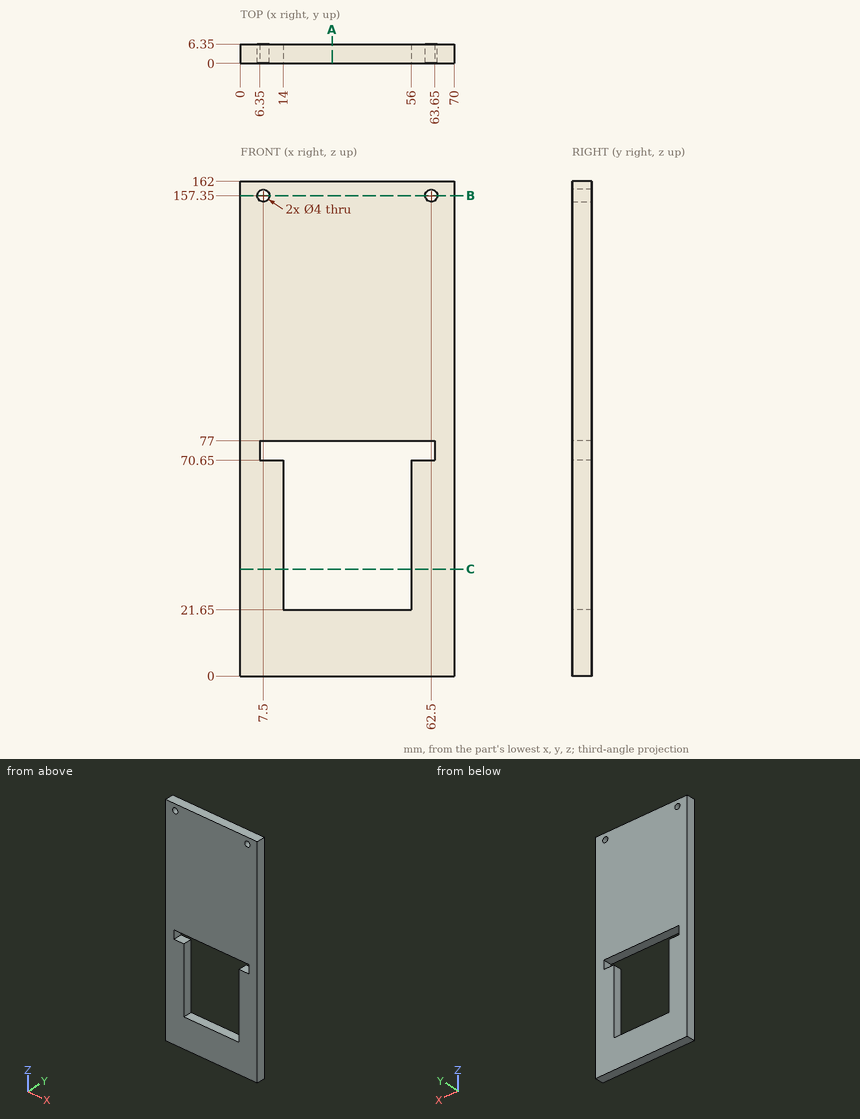
Could you check a few things on this drawing? It's one solid part, dimensions in mm from its lowest x, y, z. Round coordinates to 2 decimals unless told otherwise and drop trailing zeros. Write each loop counter-clockwise with the first axis right and the second up, starting at its lowest first coordinate (ties: lowest second). Pieces come first, ordered by that corner, then holes.
Q1. If we section it at B-B on z = 157.35: Write out the boundary of the cut face in (x, y).
Q2. If we section it at A-A on x = 30: Write out the boundary of the cut face in (y, z).
Q3. Please list where these lines run through material, in increasing order: probe 1 along X at (y, z) = (2.5, 157.35); probe 2 along Z at (x, y) = (46, 5); probe 3 along X at (y, z) = (1.5, 43).
Q4. If we section it at C-C on z = 35: Write out the boundary of the cut face in (x, y).
Q5. Will these pins go through, and if not, where does the flat tip stop? P1, Ø3, axis at x = 37.5, y = 5, coming from the -Z side; P2, Ø2.5, axis at x = 7.5, z = 157.35, coming from the -Y side.
Answer below:
1. outline: (0, 0) - (5.5, 0) - (5.5, 6.35) - (0, 6.35) - close; (9.5, 0) - (60.5, 0) - (60.5, 6.35) - (9.5, 6.35) - close; (64.5, 0) - (70, 0) - (70, 6.35) - (64.5, 6.35) - close
2. outline: (0, 0) - (6.35, 0) - (6.35, 21.65) - (0, 21.65) - close; (0, 77) - (6.35, 77) - (6.35, 162) - (0, 162) - close
3. probe 1: x = 0 to 5.5, 9.5 to 60.5, 64.5 to 70
3. probe 2: z = 0 to 21.65, 77 to 162
3. probe 3: x = 0 to 14, 56 to 70
4. outline: (0, 0) - (14, 0) - (14, 6.35) - (0, 6.35) - close; (56, 0) - (70, 0) - (70, 6.35) - (56, 6.35) - close
5. P1: stops at z = 0
5. P2: passes through
